from build123d import *

# Parameters (mm, degrees)
CHAFL_N1_SIZE = 0.5


with BuildPart() as part:
    # Croquis1 → Revolución1 (revolve)
    with BuildSketch(Plane(origin=(0, 0, 0), x_dir=(-1, 0, 0), z_dir=(0, 1, 0)), mode=Mode.PRIVATE) as revoluci_n1_sk:
        Polygon((-10.9, 3), (10.9, 3), (10.9, 2.55), (11.7, 2.55), (11.7, 3), (15.9, 3), (15.9, 0), (-15.9, 0), (-15.9, 3), (-11.7, 3), (-11.7, 2.55), (-10.9, 2.55), align=None)
    revolve(revoluci_n1_sk.sketch.rotate(Axis((15.9, 0, 0), (-1, 0, 0)), 180), axis=Axis((15.9, 0, 0), (-1, 0, 0)))

    # Chaflán1
    chafl_n1_edges = [part.edges().sort_by_distance(p)[0] for p in [
        (-15.9, 0, 3),
        (15.9, 0, 3),
    ]]
    chamfer(chafl_n1_edges, length=CHAFL_N1_SIZE)


solid = part.part
Read the model definition and answer for the solid it produces. Units are mm, in the model's axes. A direction names the side the tool comes from. Round coordinates to 2 decimals unless told otherwise and drop trailing zeros. Order: outer loops, then holes, each group sorted by start corner. A loop starts at its lowest first (then second) coordinate and runs counter-clockwise, first axis right, second up.
1) The mould has two halves that part along X. Classify faces 3 (the face through (11.29, -0.77, -2.43)), 4 (the face through (15.9, 0, 0)), 5 (the face through (13.52, -0.9, -2.86)): released by +X, released by -X, zero draft, split by the parting line, or undercut.
2) The part is cut by section A-A on x = 0. Write down the section's boundary in (y, z).
3) Straight lines are drawn through the part: L1, parallel to X at y = 1.7, z = 1.95; L2, parallel to X at y = -2.25, z = -1.45; L3, parallel to Z at x = 5, y = -0.2. For each, find the intervals that lie inside material, in ascending order.
4) For faces 1 (the face through (-13.58, -0.9, -2.86)), 2 (the face through (11.7, -2, 2)), determine the directions among +Z, -Z, +X, -X, +Y, -Y from which every point of the face is accessible in a straight line to the end or side of a thin tool.
5) A flat-ended cylindrical pin translates along its axis: pin 1 (1 mm diameter, centred on x = 7, y = -1.5, fed in from -Z). Find the tip coordinate at first contact, or state that the pin passes through.
Resolved:
1. face 3: undercut
1. face 4: released by +X
1. face 5: zero draft
2. outline: circle Ø6 at (0, 0)
3. L1: x = -15.81 to -11.7, -10.9 to 10.9, 11.7 to 15.81
3. L2: x = -15.72 to -11.7, -10.9 to 10.9, 11.7 to 15.72
3. L3: z = -2.99 to 2.99
4. face 1: +X, -X
4. face 2: none
5. pin 1: stops at z = -2.83
